```python
from build123d import *

# Parameters (mm, degrees)
CROQUIS1_W              = 42
CROQUIS1_H              = 85
CROQUIS1_R              = 2.05
SALIENTE_EXTRUIR1_DEPTH = 5
CROQUIS4_R              = 4.05
CORTAR_EXTRUIR1_DEPTH   = 2.8
CROQUIS7_R              = 5
CORTAR_EXTRUIR4_DEPTH   = 6
CROQUIS8_W              = 42
CROQUIS8_H              = 7.7
SALIENTE_EXTRUIR2_DEPTH = 5
CHAFL_N1_SIZE           = 4.1


with BuildPart() as part:
    # Croquis1 → Saliente-Extruir1 (new body)
    with BuildSketch(Plane.XY):
        with Locations((21, 42.5)):
            Rectangle(CROQUIS1_W, CROQUIS1_H)
        with Locations((11, 76.8)):
            Circle(CROQUIS1_R, mode=Mode.SUBTRACT)
        with Locations((31, 76.8)):
            Circle(CROQUIS1_R, mode=Mode.SUBTRACT)
        with Locations((31, 56.8)):
            Circle(CROQUIS1_R, mode=Mode.SUBTRACT)
        with Locations((11, 56.8)):
            Circle(CROQUIS1_R, mode=Mode.SUBTRACT)
    extrude(amount=SALIENTE_EXTRUIR1_DEPTH)

    # Croquis4 → Cortar-Extruir1 (cut)
    with BuildSketch(Plane.XY.offset(5)):
        with Locations((11, 76.8)):
            Circle(CROQUIS4_R)
        with Locations((11, 56.8)):
            Circle(CROQUIS4_R)
        with Locations((31, 56.8)):
            Circle(CROQUIS4_R)
        with Locations((31, 76.8)):
            Circle(CROQUIS4_R)
    extrude(amount=-CORTAR_EXTRUIR1_DEPTH, mode=Mode.SUBTRACT)

    # Croquis7 → Cortar-Extruir4 (cut, through all)
    with BuildSketch(Plane.XY.offset(5)):
        with Locations((21, 21.08)):
            Circle(CROQUIS7_R)
    extrude(amount=-CORTAR_EXTRUIR4_DEPTH, mode=Mode.SUBTRACT)

    # Croquis8 → Saliente-Extruir2 (add, through all)
    with BuildSketch(Plane.XY.offset(5)):
        with Locations((21, -3.85)):
            Rectangle(CROQUIS8_W, CROQUIS8_H)
    extrude(amount=-SALIENTE_EXTRUIR2_DEPTH)

    # Chaflán1
    chafl_n1_edges = [part.edges().sort_by_distance(p)[0] for p in [
        (0, -7.7, 2.5),
        (42, -7.7, 2.5),
    ]]
    chamfer(chafl_n1_edges, length=CHAFL_N1_SIZE)


solid = part.part
```
Work out the finished part from the listing and answer in its coordinate system (mm). A direction names the side the tool comes from. Give positions to 0.01 mm unless a question says otherwise; leave off trailing zeros. Loops run counter-clockwise (first coordinate to the right, second up) from the corner with the lowest first, then second, coordinate; pieces in that order, holes last. Notation, with made-up numbers: M -1,-23 L 27,-23 A9 ccw 27,-12 Z; hole C 38.5,44.25 d7. An arc over 180 degrees is marked long. One line per item, written item: value. Start each with the question number.
1. Determine the mould class of faces 1 (the face through (42, 40, 3)), 2 (the face through (21, -7.7, 3)), 3 (the face through (10.733, 78.833, 1.085)) for opening direction Y: released by +Y, released by -Y, zero draft, split by the parting line, or undercut.
2. Each of these flat-tipped pins is pushed along its axis until it touches: P1, Ø6.5, axis at x = 11, y = 76.8, coming from the +Z side; P2, Ø3.5, axis at x = 31, y = 56.8, coming from the +Z side. Where does it stop, or does it pass through?
3. Which of the six approach directions +Z, -Z, +X, -X, +Y, -Y give full straight-line access (tool end or side, diameter ignored) to faces 4 (the face through (30, 79, 2.2)), 5 (the face through (21, 39, 5))?
4. Find section B-B (y = 76.8). Give the vertices of the cut face in (x, z).
5. Find section D-D (x = 11). Give the vertices of the cut face in (y, z).
6. Find section A-A (x = 21). Give the vertices of the cut face in (y, z).
7. Find the intervals of material crossed by probe 1 along X at (y, z) = (56.8, 1); probe 2 along Y at (x, z) = (31, 1.5); probe 3 along Y at (x, z) = (11, 4.2), in increasing order.
8. Find section C-C (z = 3.45). Give the vertices of the cut face in (x, y).
Reported:
1. face 1: zero draft
1. face 2: released by -Y
1. face 3: undercut
2. P1: stops at z = 2.2
2. P2: passes through
3. face 4: +Z
3. face 5: +Z, +X, -X, +Y, -Y
4. outline: M 0,0 L 8.95,0 L 8.95,2.2 L 6.95,2.2 L 6.95,5 L 0,5 Z; M 13.05,0 L 28.95,0 L 28.95,2.2 L 26.95,2.2 L 26.95,5 L 15.05,5 L 15.05,2.2 L 13.05,2.2 Z; M 33.05,0 L 42,0 L 42,5 L 35.05,5 L 35.05,2.2 L 33.05,2.2 Z
5. outline: M -7.7,0 L 54.75,0 L 54.75,2.2 L 52.75,2.2 L 52.75,5 L -7.7,5 Z; M 58.85,0 L 74.75,0 L 74.75,2.2 L 72.75,2.2 L 72.75,5 L 60.85,5 L 60.85,2.2 L 58.85,2.2 Z; M 78.85,0 L 85,0 L 85,5 L 80.85,5 L 80.85,2.2 L 78.85,2.2 Z
6. outline: M -7.7,0 L 16.08,0 L 16.08,5 L -7.7,5 Z; M 26.08,0 L 85,0 L 85,5 L 26.08,5 Z
7. probe 1: x = 0 to 8.95, 13.05 to 28.95, 33.05 to 42
7. probe 2: y = -7.7 to 54.75, 58.85 to 74.75, 78.85 to 85
7. probe 3: y = -7.7 to 52.75, 60.85 to 72.75, 80.85 to 85
8. outline: M 0,-3.6 L 4.1,-7.7 L 37.9,-7.7 L 42,-3.6 L 42,85 L 0,85 Z; hole C 11,56.8 d8.1; hole C 11,76.8 d8.1; hole C 21,21.08 d10; hole C 31,56.8 d8.1; hole C 31,76.8 d8.1
